For this review, take the finished solid that the model builds, in its own axes (mm). A direction names the side the tool comes from. Round coordinates to 2 decimals unless told otherwise and drop trailing zeros. Loops run counter-clockwise (first coordinate to the right, second up) from the corner with the lowest first, then second, coordinate; pieces in that order, holes last. Notation, with made-up numbers: (-12, 26.5) -> (40, 26.5) arc R18 ccw to (40, 51.5) -> close; hole circle Ø9 at (-18, -12). An arc over 180 degrees is marked (long way). One line per question, with ' | ' between items. Start each with the question number.
1. Draft analysis for pull direction Y (two halves, no side actions). For faces 1 (the face through (20, 5, -19)), 2 (the face through (14.08, 6.2, -18.16)), 3 (the face through (10, 29, -20)), state which applies: pulls with the +Y half, pulls with the -Y half, needs draft (parallel to the pull), parting line crosses it, or undercut.
2. Consider section D-D (x = 16). Write out the cut boundary in (y, z).
3. Consider section A-A (z = 10). Write out the cut boundary in (x, y).
4. Consider section C-C (y = 13). Write out the cut boundary in (x, z).
5. For faces 4 (the face through (10, 3, 20)), 5 (the face through (3.944, 15.884, -30.913)), list the 3-axis set-ups (+Z, -Z, +X, -X, +Y, -Y) from which the entire face can be reached by the end or side of a thin tool; tool diameter is ignored.
6. Consider section B-B (x = 10.5). Write out the cut boundary in (y, z), and give its area (3 significant figures).
7. For pin 1 Ø6.5 at (x, z) = (10, 10) entering from +Y; pin 2 Ø4.5 at (x, z) = (10, -50) entering from +Y; pin 3 Ø12 at (x, y) = (3, 23.5) entering from -Z; pin 4 Ø3 at (x, z) = (10, -27.5) entering from +Y, all flat-tipped, find the tip position at first contact; note any pin that passes through.
8. Wall thickness on line 1 along X through (y, z) = (1, -50); line 2 along Y through (x, z) = (16.5, -20); line 3 along Z through (x, y) = (10, 3.85): over which ranges is each line inside the solid? List them lowest first.
Autodesk Inventor part; units mm, degrees
ref_plane "YZ Plane" through (0, 0, 0) normal (1, 0, 0) x (0, 1, 0)
ref_plane "XZ Plane" through (0, 0, 0) normal (0, 1, 0) x (-1, 0, 0)
ref_plane "XY Plane" through (0, 0, 0) normal (0, 0, 1) x (1, 0, 0)
sketch "Sketch1" plane through (0, 0, 0) normal (1, 0, 0) x (0, 1, 0)
  line L0 (0, 0) -> (5, 0)
  line L1 (5, 0) -> (5, -40)
  line L2 (5, -40) -> (0, -40)
  line L3 (0, -40) -> (0, 0)
  line L4 (5, -20) -> (10.5, -20)
  circle A0 centre (10.5, -20) radius 4
  line L5 (10.5, -16) -> (5, -16)
  line L6 (10.5, -24) -> (5, -24)
  circle A1 centre (10.5, -20) radius 5.5
  line L7 (14.277, -16.0019) -> (5, -7.2379)
  line L8 (14.2701, -24.0045) -> (5, -32.7321)
  dimension "d0" = 5
  dimension "d1" = 40
  dimension "d2" = 5.5
  dimension "d3" = 8
extrude "Extrusion1" add sketch "Sketch1" along normal blind 20 contours L0 L1 L2 L3 | L7 A1 L5 L1 | L5 A1 L1 | A1 L6 A0 L5 | L1 L6 A1 L8 | A1 L6 L1 | A1 L5 A0 L4 | L4 A0 L6 A1
sketch "Sketch2" plane through (0, 0, -40) normal (0, 0, -1) x (-1, 0, 0)
  line L0 (0, 5) -> (-20, 5)
  line L1 (-20, 5) -> (0, 5)
  line L2 (0, 5) -> (0, 0)
  line L3 (0, 0) -> (-20, 0)
  line L4 (-20, 0) -> (-20, 5)
extrude "Extrusion2" add sketch "Sketch2" along normal blind 20
sketch "Sketch3" plane through (0, 0, 0) normal (0, 0, 1) x (1, 0, 0)
  line L0 (0, 5) -> (20, 5)
  line L1 (20, 5) -> (20, 0)
  line L2 (0, 5) -> (20, 5)
  line L3 (20, 5) -> (20, 0)
  line L4 (20, 0) -> (0, 0)
  line L5 (0, 0) -> (0, 5)
extrude "Extrusion3" add sketch "Sketch3" along normal blind 20
fillet "Fillet1" radius 4 2 edges at (10, 5, -32.7321) (10, 5, -7.2379)
sketch "Sketch4" plane through (0, 5, 20) normal (0, 1, 0) x (1, 0, 0)
  line L0 (0, 80) -> (0, 0)
  line L1 (0, 0) -> (10, 0)
  line L2 (0, 0) -> (20, 0)
  line L3 (10, 0) -> (10, 10)
  circle A0 centre (10, 10) radius 2.5
  line L4 (0, 80) -> (10, 80)
  line L5 (0, 80) -> (20, 80)
  line L6 (10, 80) -> (10, 70)
  circle A1 centre (10, 70) radius 2.5
  point P0 (0, 20)
  dimension "d11" = 10
  dimension "d12" = 10
  dimension "d13" = 5
  dimension "d14" = 10
  dimension "d15" = 5
extrude "Extrusion4" cut sketch "Sketch4" against normal blind 20
sketch "Sketch5" plane through (20, 0, 0) normal (1, 0, 0) x (0, 0, -1)
  circle A0 centre (20, 10.5) radius 4
  circle A1 centre (20, 10.5) radius 7
  line L0 (16, 16.2446) -> (0, 5)
  line L1 (5.5141, 5) -> (-20, 5)
  line L2 (34.46, 5) -> (60, 5)
  line L3 (20, 17.5) -> (20, 10.5)
  line L4 (24, 16.2446) -> (40, 5)
  line L5 (40, 5) -> (24.3301, 5)
  line L6 (0, 5) -> (15.6699, 5)
  point P0 (0, 0)
  point P1 (40, 5)
  dimension "d18" = 14
extrude "Extrusion5" add sketch "Sketch5" against normal blind 20
fillet "Fillet2" radius 4 2 edges at (10, 5, -40) (10, 5, 0)
sketch "Sketch6" plane through (0, 0, 0) normal (-1, 0, 0) x (0, 0, 1)
  circle A0 centre (-20, 10.5) radius 4
  line L0 (-20, 10.5) -> (-20, 14.5)
  circle A1 centre (-20, 14.5) radius 11
  circle A2 centre (-20, 14.5) radius 14.5
  arc A3 (-41.265, 5) -> (-38.965, 5.7274) centre (-41.265, 9) ccw
  line L1 (-41.265, 5) -> (-32.8706, 21.1782)
  line L2 (1.265, 5) -> (20, 5)
  line L3 (1.265, 5) -> (-7.1294, 21.1782)
  line L4 (-41.265, 5) -> (-23.6138, 0.4575)
  arc A4 (-1.035, 5.7274) -> (1.265, 5) centre (1.265, 9) ccw
  line L5 (-16.3862, 0.4575) -> (1.265, 5)
  point P0 (0, 0)
  dimension "d23" = 4
  dimension "d24" = 22
extrude "Extrusion6" add sketch "Sketch6" against normal blind 20 contours A2 | A2 L3 L5 | A2 L4 L1
sketch "Sketch7" plane through (0, 0, 0) normal (-1, 0, 0) x (0, 0, 1)
  circle A0 centre (-20, 10.5) radius 4
  circle A1 centre (-20, 14.5) radius 11
  point P0 (0, 0)
extrude "Extrusion7" cut sketch "Sketch7" against normal blind 20
fillet "Fillet3" radius 4 2 edges at (10, 5, -41.265) (10, 5, 1.265)
sketch "Sketch8" plane through (0, 5, 20) normal (0, 1, 0) x (1, 0, 0)
  circle A0 centre (10, 10) radius 2.5
  circle A1 centre (10, 10) radius 7.4
  circle A2 centre (10, 70) radius 2.5
  circle A3 centre (10, 70) radius 7.4
  point P0 (0, 20)
  dimension "d30" = 14.8
  dimension "d31" = 14.8
extrude "Extrusion8" cut sketch "Sketch8" along normal blind 10
sketch "Sketch9" plane through (20, 0, 0) normal (1, 0, 0) x (0, 0, -1)
  circle A0 centre (20, 14.5) radius 11
  circle A1 centre (20, 14.5) radius 11
  circle A2 centre (20, 14.5) radius 8.5
  point P0 (0, 0)
  dimension "d34" = 17
extrude "Extrusion9" add sketch "Sketch9" against normal blind 12
properties part number "base_axis_8mm_2020" material "PET Plastic"
Answer block:
1) face 1: needs draft | face 2: undercut | face 3: pulls with the +Y half
2) outline: (0, -60) -> (5, -60) -> (5, -43.7) arc R4 cw to (7.16, -40.15) -> (21.18, -32.87) arc R14.5 ccw to (21.18, -7.13) -> (7.16, 0.15) arc R4 cw to (5, 3.7) -> (5, 20) -> (0, 20) -> close; hole circle Ø17 at (14.5, -20)
3) outline: (0, 0) -> (7.5, 0) -> (7.5, 5) -> (0, 5) -> close; (12.5, 0) -> (20, 0) -> (20, 5) -> (12.5, 5) -> close
4) outline: (0, -37.11) -> (20, -37.11) -> (20, -28.37) -> (8, -28.37) -> (8, -30.9) -> (0, -30.9) -> close; (0, -9.1) -> (8, -9.1) -> (8, -11.63) -> (20, -11.63) -> (20, -2.89) -> (0, -2.89) -> close
5) face 4: +Z, +X, -X, +Y, -Y | face 5: -X
6) outline: (0, -60) -> (5, -60) -> (5, -52.45) -> (0, -52.45) -> close; (0, -47.55) -> (5, -47.55) -> (5, -42.62) -> (5.15, -42.62) arc R4 cw to (7.16, -40.15) -> (21.18, -32.87) arc R14.5 ccw to (21.18, -7.13) -> (7.16, 0.15) arc R4 cw to (5.15, 2.62) -> (5, 2.62) -> (5, 7.55) -> (0, 7.55) -> close; (0, 12.45) -> (5, 12.45) -> (5, 20) -> (0, 20) -> close; hole circle Ø17 at (14.5, -20) | area: 822 mm2
7) pin 1: stops at y = 5 | pin 2: passes through | pin 3: stops at z = -34.78 | pin 4: stops at y = 27.7
8) line 1: x = 0 to 7.5, 12.5 to 20 | line 2: y = 0 to 6, 23 to 29 | line 3: z = -60 to -52.5, -47.5 to 7.5, 12.5 to 20
